Check sheet for the modelled part. Datum: model origin and axes. Units: mm. A direction names the side the tool comes from. Give positions to 0.01 mm unless a question says otherwise; leave off trailing zeros. Write each loop counter-clockwise with the first axis right and the second up, starting at its lowest first coordinate (ties: lowest second). Pieces come first, ordered by that corner, then holes. Notation, with made-up numbers: M 81,66.25 L 86,66.25 A25 cw 86,103.25 Z; hole C 30,78 d4. An arc over 180 degrees is marked long. One line per item, written item: value. Start each with the question number.
from build123d import *

# Parameters (mm, degrees)
SKETCH1_W              = 125
SKETCH1_H              = 15
SKETCH1_W_2            = 115.16
SKETCH1_H_2            = 5
SLIDER_MAIN_BODY_DEPTH = 5
SKETCH5_W              = 105.16
SKETCH5_H              = 1.666666666
CUT_EXTRUDE1_DEPTH     = 65.468984791
SKETCH6_W              = 115.16
SKETCH6_H              = 5
CUT_EXTRUDE2_DEPTH     = 64.146654702


with BuildPart() as part:
    # Sketch1 → Slider Main Body (new body)
    with BuildSketch(Plane.XY):
        Rectangle(SKETCH1_W, SKETCH1_H)
        Rectangle(SKETCH1_W_2, SKETCH1_H_2, mode=Mode.SUBTRACT)
    extrude(amount=SLIDER_MAIN_BODY_DEPTH)

    # Sketch5 → Cut-Extrude1 (cut, through all)
    with BuildSketch(Plane.XZ.offset(7.5)):
        with Locations((0, 2.5)):
            Rectangle(SKETCH5_W, SKETCH5_H)
    extrude(amount=-CUT_EXTRUDE1_DEPTH, mode=Mode.SUBTRACT)

    # Sketch6 → Cut-Extrude2 (cut, through all)
    with BuildSketch(Plane.XY.offset(5)):
        with Locations((0, 5)):
            Rectangle(SKETCH6_W, SKETCH6_H)
    extrude(amount=-CUT_EXTRUDE2_DEPTH, mode=Mode.SUBTRACT)


solid = part.part
1) Cross-section at C-C (y = -4.75). Record the boundary of the cut face in (x, z).
2) Cross-section at D-D (z = 4.1). Record the boundary of the cut face in (x, y).
3) Cross-section at B-B (x = 4.5). Record the boundary of the cut face in (y, z), plus the area to 3 significant figures.
4) Draft check along X on faces 1 (the flat face through (-1, -7.5, 1)), 2 (the flat face through (-1, -5, 1.667)), 3 (the flat face through (-62.5, 0, 2)). Enter one of: released by +X, released by -X, zero draft, split by the parting line, or undercut.
5) Cross-section at A-A (y = 3.75). Record the boundary of the cut face in (x, z), plus the area to 3 significant figures.
6) Material ranges on L1, parallel to X at y = 4.75, z = 4.3; L2, parallel to Z at x = 6, y = -3; L3, parallel to Y at x = 19, z = 3.6, recorded low to high. Write a range as from..to.
7) Tool access check on faces 4 (the flat face through (0, -4, 0)), 5 (the flat face through (-1, -2.5, 1)), 6 (the flat face through (-1, -5, 3.333)). Record the directions out of +Z, -Z, +X, -X, +Y, -Y that give a thin tool (end or side, any length) a straight path to the whole face; none if there is none.
Data:
1. outline: M -62.5,0 L 62.5,0 L 62.5,5 L -62.5,5 Z; hole M -52.58,1.67 L 52.58,1.67 L 52.58,3.33 L -52.58,3.33 Z
2. outline: M -62.5,-7.5 L 62.5,-7.5 L 62.5,7.5 L 57.58,7.5 L 57.58,-2.5 L -57.58,-2.5 L -57.58,7.5 L -62.5,7.5 Z
3. outline: M -7.5,0 L -2.5,0 L -2.5,1.67 L -7.5,1.67 Z; M -7.5,3.33 L -2.5,3.33 L -2.5,5 L -7.5,5 Z
3. area: 16.7 mm2
4. face 1: zero draft
4. face 2: undercut
4. face 3: released by -X
5. outline: M -62.5,0 L -57.58,0 L -57.58,5 L -62.5,5 Z; M 57.58,0 L 62.5,0 L 62.5,5 L 57.58,5 Z
5. area: 49.2 mm2
6. L1: x = -62.5..-57.58, 57.58..62.5
6. L2: z = 0..1.67, 3.33..5
6. L3: y = -7.5..-2.5
7. face 4: -Z, +X, -X, +Y, -Y
7. face 5: +Z, -Z, +Y
7. face 6: +Y, -Y
